The figure shows three views and two pictorial views of one solid part (mm, origin at its lowest corner). Answer the questions. A direction names the side the tool comes from. Coordinates: 2 decimals unless noted, no trailing zeros. Order: outer loops, then holes, each group sorted by start corner. A loop starts at its lowest first (then second) coordinate and runs counter-clockwise, first axis right, second up.
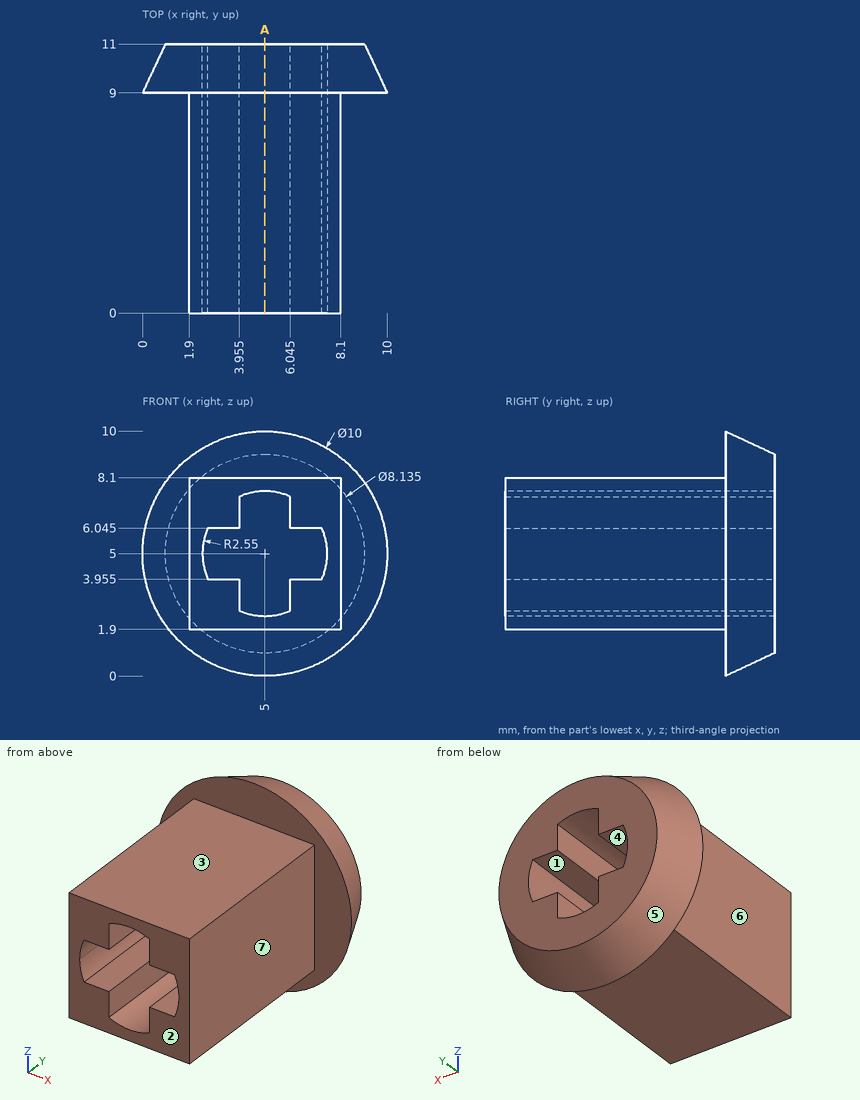
1) The mould has two halves that part along X. Classify the marked faces 4, 5, 6 and 7: released by +X, released by -X, zero draft, split by the parting line, or undercut.
2) For the marked faces 1, 2 and 3, determine the directions among +Z, -Z, +X, -X, +Y, -Y from which every point of the face is accessible in a straight line to the end or side of a thin tool.
3) Straight lines are drawn through the part: probe 1 along Z at (x, y) = (3.5, 1.75) (3 decimals); probe 2 along X at (y, z) = (6.25, 5); probe 3 along Z at (x, y) = (8, 1). For each, find the intervals that lie inside material, in ascending order.
4) Each of these flat-tipped pins is pushed along its axis until it touches: P1, Ø1.4, axis at x = 7, y = 5, coming from the -Z side; P2, Ø0.6, axis at y = 3, z = 6.5, coming from the +X side; P3, Ø1.9, axis at x = 4.5, y = 6, coming from the +Z side. Where does it stop, or does it pass through?
5) A cutting plane is placed at A-A, the plane x = 5. Write down the section's boundary in (y, z).
Working result:
1. face 4: undercut
1. face 5: split by the parting line
1. face 6: released by -X
1. face 7: released by +X
2. face 1: +Y, -Y
2. face 2: +Z, -Z, +X, -X, -Y
2. face 3: +Z, +X, -X, -Y
3. probe 1: z = 1.9 to 3.955, 6.045 to 8.1
3. probe 2: x = 1.9 to 2.45, 7.55 to 8.1
3. probe 3: z = 1.9 to 8.1
4. P1: stops at z = 1.9
4. P2: stops at x = 8.1
4. P3: stops at z = 8.1
5. outline: (0, 1.9) - (9, 1.9) - (9, 0) - (11, 0.93) - (11, 2.45) - (0, 2.45) - close; (0, 7.55) - (11, 7.55) - (11, 9.07) - (9, 10) - (9, 8.1) - (0, 8.1) - close
